Geometry check sheet. Reference: the model listing, model coordinates, mm. Give positions to 0.01 mm unless a question says otherwise; leave off trailing zeros. Loops run counter-clockwise (first coordinate to the right, second up) from the corner with the lowest first, then second, coordinate; pieces in that order, holes last. Notation, with made-up numbers: (39, -30.75) -> (52, -30.75) arc R26 ccw to (52, -12.75) -> close; hole circle Ø2 at (57, 10.25). An arc over 180 degrees is marked (long way). One line per item, written item: value. Start each with the question number.
(1) Scan lines: line 1 along X through (y, z) = (-3.5, 1.55); line 2 along X through (y, z) = (3, 0.4); line 3 along Y through (x, z) = (9.5, 1.2). Record each from-to range of solid material in increasing order. Write a range as from..to.
(2) Gauge pin test, flat ends, axial feed: pin 1 Ø1 at (y, z) = (11.5, 1) entering from +X; pin 2 Ø1 at (x, y) = (1, 18) entering from -Z. Record the tip position at first contact, or that the pin passes through.
(3) Sectioned sample at A-A, the plane x = 0. Record the cut outline in (y, z) (3 decimals), then the cut area to 3 significant figures.
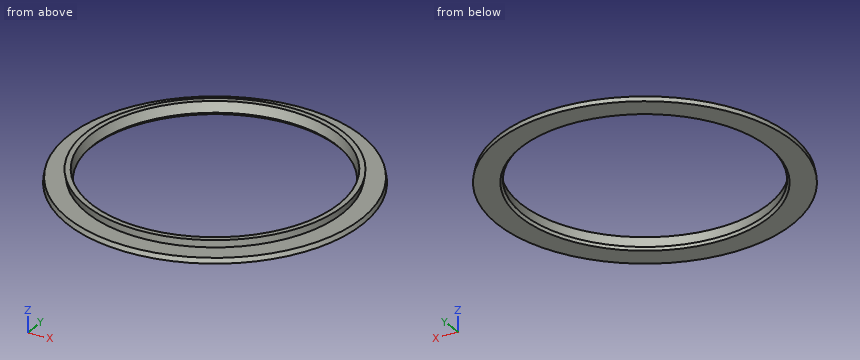
from build123d import *

# Parameters (mm, degrees)
F0_R     = 22.65
F0_R_2   = 18.65
F1_DEPTH = 2
F1_TAPER = 10
F2_T     = -0.8


# Not quite as in the source:
# - a fillet or chamfer that OpenCascade refuses, or shapes differently, is made with other operations: its cross-section is extruded or revolved along the edge and cut away or added


with BuildPart() as f1:
    # F0 (on Top) → F1 (new body)
    with BuildSketch(Plane.XY):
        Circle(F0_R)
        Circle(F0_R_2, mode=Mode.SUBTRACT)
    extrude(amount=F1_DEPTH, taper=F1_TAPER)

    # F2
    f2_openings = [f1.faces().sort_by_distance(p)[0] for p in [
        (-21.666682, 0, 2),
        (-22.473673, 0, 1),
    ]]
    offset(amount=F2_T, openings=f2_openings, kind=Kind.INTERSECTION)

    # F3: chamfer of 0.4 on 1 edges, made by hand

    # F3_s1 → F3_t2 (revolve, cut)
    with BuildSketch(Plane.XZ):
        Polygon((18.7194592711, 0.3939231012), (19.05, 0), (18.65, 0), align=None)
    revolve(axis=Axis((0, 0, 0), (0, 0, 1)), mode=Mode.SUBTRACT)


solid = f1.part
Calculated:
1. line 1: x = -19.42..-18.6, 18.6..19.42
1. line 2: x = -22.38..-18.48, 18.48..22.38
1. line 3: y = -17.23..-16.29, 16.29..17.23
2. pin 1: stops at x = 19.61
2. pin 2: passes through
3. outline: (-22.65, 0) -> (-19.05, 0) -> (-18.719, 0.394) -> (-19.003, 2) -> (-19.815, 2) -> (-19.603, 0.8) -> (-22.509, 0.8) -> close; (18.719, 0.394) -> (19.05, 0) -> (22.65, 0) -> (22.509, 0.8) -> (19.603, 0.8) -> (19.815, 2) -> (19.003, 2) -> close
3. area: 7.97 mm2
